Input: dimensioned drawing with shaded views. Units: mm. Origin: part minimum x, y, z. A direction names the side the tool comes from. Coordinates: 2 decimals unless noted, no trailing zeros. Write each loop counter-clockwise with the first axis right and the second up, starting at its lowest first coordinate (ties: lowest second). Pieces come first, ordered by that corner, then holes. Notation, with made-up numbers: (-26.5, 19.5) -> (-4.5, 19.5) arc R33 ccw to (-4.5, 53.5) -> close; hole circle Ø6 at (52, -21). An arc over 180 degrees is marked (long way). One line per item, written item: value. Start each with the question number.
1. Mould query, pull axis Z, two halves, no side actions, for the marked faces 1, 2 and 3. Classes: released by +Z, released by -Z, zero draft, split by the parting line, or undercut.
2. First-contact query: P1, Ø2, axis at y = 5.5, z = 0.5, coming from the +X side (3 decimals); P2, Ø2, axis at x = 1.5, y = 6, coming from the -Z side; P3, Ø12, axis at x = 32.5, z = 12, coming from the -Y side; P4, Ø2, axis at y = 7, z = 14, coming from the -X side. Flat tips, straight axial feed; report the tip coordinate or a pass-through.
3. Section query D-D, the plane y = 7. Output: boundary loops of the cut face in (x, z) (1 decimal), and give its area (3 significant figures).
4. Section query C-C, the plane z = 4.25. Output: boundary loops of the cut face in (x, y).
5. Section query A-A, the plane z = 17. Output: boundary loops of the cut face in (x, y) (1 decimal).
6. Line query: line 1 (X direction, y = 6.75, z = 12.25); line 2 (X direction, y = 7.25, z = 18) (1 decimal); line 3 (Z direction, x = 24, y = 1.75). Output: solid intervals per line, ascending.
7. Access query for the marked faces 4 and 5. Directions: +Z, -Z, +X, -X, +Y, -Y. A direction counts if a zero-diameter tool reaches every point of the face in a straight line with its end or side. Return the directions, or none.
8. Section query B-B, the plane x = 41. Output: boundary loops of the cut face in (y, z) (3 decimals).
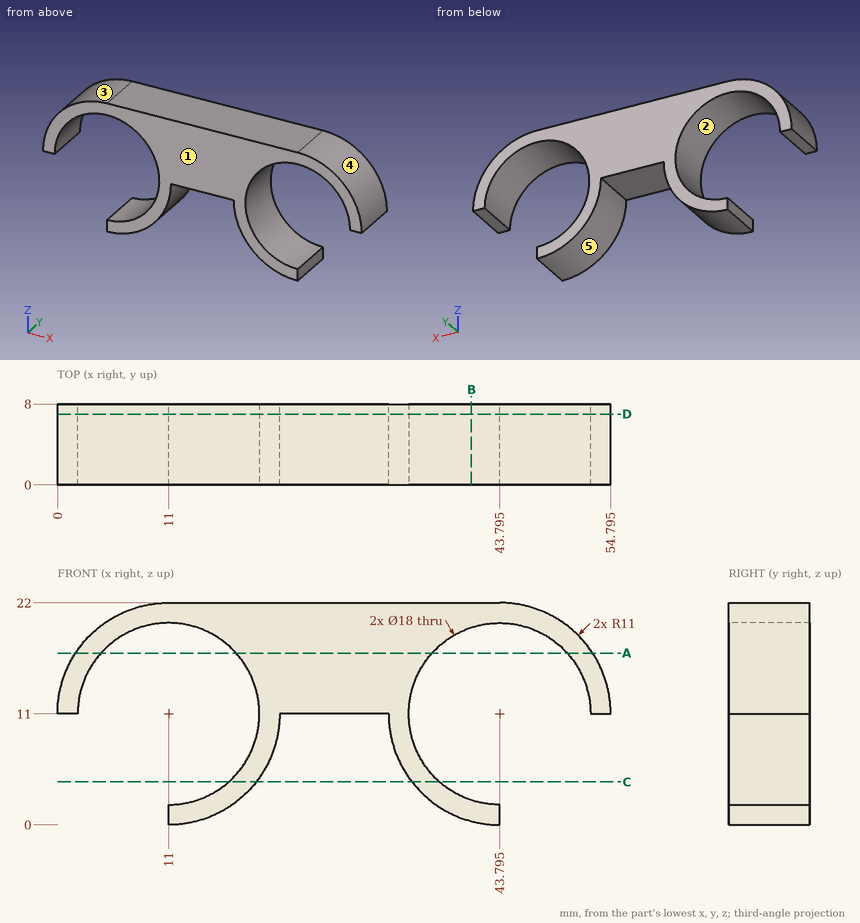
Computed values:
1. face 1: zero draft
1. face 2: undercut
1. face 3: released by +Z
2. P1: stops at x = 43.795
2. P2: stops at z = 11
2. P3: stops at y = 0
2. P4: stops at x = 0.18
3. outline: (0, 11) -> (2, 11) arc R9 cw (long way) to (11, 2) -> (11, 0) arc R11 ccw to (22, 11) -> (32.8, 11) arc R11 ccw to (43.8, 0) -> (43.8, 2) arc R9 cw (long way) to (52.8, 11) -> (54.8, 11) arc R11 ccw to (43.8, 22) -> (11, 22) arc R11 ccw to start
3. area: 359 mm²
4. outline: (16.95, 0) -> (19.69, 0) -> (19.69, 8) -> (16.95, 8) -> close; (35.11, 0) -> (37.84, 0) -> (37.84, 8) -> (35.11, 8) -> close
5. outline: (1.8, 0) -> (4.3, 0) -> (4.3, 8) -> (1.8, 8) -> close; (17.7, 0) -> (37.1, 0) -> (37.1, 8) -> (17.7, 8) -> close; (50.5, 0) -> (53, 0) -> (53, 8) -> (50.5, 8) -> close
6. line 1: x = 0.07 to 2.09, 19.91 to 34.88, 52.71 to 54.72
6. line 2: x = 2.5 to 5.3, 16.7 to 38.1, 49.5 to 52.3
6. line 3: z = 11 to 22
7. face 4: +Z, +X, +Y, -Y
7. face 5: -Z, +Y, -Y
8. outline: (0, 0.361) -> (8, 0.361) -> (8, 2.445) -> (0, 2.445) -> close; (0, 19.555) -> (8, 19.555) -> (8, 22) -> (0, 22) -> close
